from build123d import *

# Parameters (mm, degrees)
F1_DEPTH = 25
F2_R     = 4
F3_DEPTH = 10
F4_R     = 10
F5_DEPTH = 25


with BuildPart() as f1:
    # F0 (on Front) → F1 (new body)
    with BuildSketch(Plane.XZ):
        Polygon((-400, 0), (0, 0), (0, 250), align=None)
        Polygon((-260.528151, 40), (-40, 177.830094), (-40, 40), align=None, mode=Mode.SUBTRACT)
    extrude(amount=F1_DEPTH)

    # F2 (on Right) → F3 (cut)
    with BuildSketch(Plane.YZ):
        with Locations((-12.5, 235)):
            Circle(F2_R)
        with Locations((-12.5, 215)):
            Circle(F2_R)
    extrude(amount=-F3_DEPTH, mode=Mode.SUBTRACT)

    # F4 (on face) → F5 (cut, through all)
    with BuildSketch(Plane.XZ.offset(25)):
        with Locations((-20, 20)):
            Circle(F4_R)
    extrude(amount=-F5_DEPTH, mode=Mode.SUBTRACT)


solid = f1.part
Check sheet for the modelled part. Datum: model origin and axes. Units: mm. A direction names the side the tool comes from. Give positions to 0.01 mm unless a question says otherwise; leave off trailing zeros. Write each loop counter-clockwise with the first axis right and the second up, starting at its lowest first coordinate (ties: lowest second). Pieces come first, ordered by that corner, then holes. Notation, with made-up numbers: (63.5, 66.25) -> (83.5, 66.25) arc R21 ccw to (83.5, 79.25) -> close; hole circle Ø4 at (-8.75, 30). An arc over 180 degrees is marked (long way). Write item = value, one per line.
Item 1: Sectioned sample at C-C on x = -20. Record the boundary of the cut face in (y, z).
Output:
outline = (-25, 0) -> (0, 0) -> (0, 10) -> (-25, 10) -> close; (-25, 30) -> (0, 30) -> (0, 237.5) -> (-25, 237.5) -> close
Item 2: Release check for a two-part mould opening along X. For faces 1 (the cylindrical face through (-10.46, -12.68, 23)), 2 (the flat face through (0, -12, 123)), 3 (the flat face through (-156, 0, 107)), 4 (the flat face through (-40, -12, 110)) record: +X half, -X half, draft (parallel to the pull), parting line (faces both ways), or undercut.
Output:
face_1 = undercut
face_2 = +X half
face_3 = draft
face_4 = undercut
Item 3: Sectioned sample at A-A on y = -12.5. Record the boundary of the cut face in (x, z).
Output:
outline = (-400, 0) -> (0, 0) -> (0, 211) -> (-10, 211) -> (-10, 219) -> (0, 219) -> (0, 231) -> (-10, 231) -> (-10, 239) -> (0, 239) -> (0, 250) -> close; hole (-260.53, 40) -> (-40, 40) -> (-40, 177.83) -> close; hole circle Ø20 at (-20, 20)
Item 4: Gauge pin test, flat ends, axial feed: pin 1 (3 mm diameter, centred on y = -3.5, z = 213.5, fed in from -X); pin 2 (18 mm diameter, centred on x = -20, z = 20, fed in from -Y) (1 decimal); pin 3 (8 mm diameter, centred on y = -16.5, z = 134.5, fed in from +X); pin 4 (7.5 mm diameter, centred on y = -12, z = 126.5, fed in from -X). Record the tip position at first contact, or that the pin passes through.
Output:
pin_1 = -60.8
pin_2 = through
pin_3 = 0
pin_4 = -203.6
Item 5: Tool access check on faces 5 (the cylindrical face through (-4.93, -13.021, 218.966)), 6 (the flat face through (-151.81, -12.32, 107.95)), 7 (the flat face through (-203, -12, 0)). Record the directions out of +Z, -Z, +X, -X, +Y, -Y that give a thin tool (end or side, any length) a straight path to the whole face; none if there is none.
Output:
face_5 = +X
face_6 = +Y, -Y
face_7 = -Z, +X, -X, +Y, -Y
Item 6: Sectioned sample at B-B on z = 20. Record the boundary of the cut face in (x, y), and give its area (3 significant figures).
Output:
outline = (-368, -25) -> (-30, -25) -> (-30, 0) -> (-368, 0) -> close; (-10, -25) -> (0, -25) -> (0, 0) -> (-10, 0) -> close
area = 8,700 mm^2
Item 7: Sectioned sample at D-D on z = 215. Record the boundary of the cut face in (x, y), and give its area (3 significant figures).
Output:
outline = (-56, -25) -> (0, -25) -> (0, -16.5) -> (-10, -16.5) -> (-10, -8.5) -> (0, -8.5) -> (0, 0) -> (-56, 0) -> close
area = 1,320 mm^2
Item 8: Scan lines: probe 1 along Z at (x, y) = (-4.75, -12.5); probe 2 along Z at (x, y) = (-233.5, -5); probe 3 along Z at (x, y) = (-20, -16.5). Record each from-to range of solid material in increasing order. Write a range as from..to.
Output:
probe_1 = 0..211, 219..231, 239..247.03
probe_2 = 0..40, 56.89..104.06
probe_3 = 0..10, 30..237.5
